```python
from build123d import *

# Parameters (mm, degrees)
SCHIZZO1_R                   = 55
ESTRUSIONE_ESTRUSIONE1_DEPTH = 47
SCHIZZO2_R                   = 51
TAGLIO_ESTRUSIONE1_DEPTH     = 44
SCHIZZO3_W                   = 6.7
SCHIZZO3_H                   = 21
ESTRUSIONE_ESTRUSIONE2_DEPTH = 25
SCHIZZO9_R                   = 1.75
TAGLIO_ESTRUSIONE2_DEPTH     = 12
TAGLIO_ESTRUSIONE3_START     = 45
SCHIZZO10_W                  = 12
SCHIZZO10_H                  = 6
TAGLIO_ESTRUSIONE3_DEPTH     = 67
SCHIZZO12_R                  = 2.2
TAGLIO_ESTRUSIONE4_DEPTH     = 90.364422451
SCHIZZO13_R                  = 4.5
ESTRUSIONE_ESTRUSIONE4_DEPTH = 44
SCHIZZO14_R                  = 1.25
TAGLIO_ESTRUSIONE6_DEPTH     = 12


with BuildPart() as part:
    # Schizzo1 → Estrusione-Estrusione1 (new body)
    with BuildSketch(Plane(origin=(0, 0, 0), x_dir=(1, 0, 0), z_dir=(0, 1, 0))):
        with Locations(Location((0, 0, 0), (0, 0, 270))):
            Circle(SCHIZZO1_R)
    extrude(amount=ESTRUSIONE_ESTRUSIONE1_DEPTH)

    # Schizzo2 → Taglio-Estrusione1 (cut)
    with BuildSketch(Plane(origin=(0, 47, 0), x_dir=(1, 0, 0), z_dir=(0, 1, 0))):
        with Locations(Location((0, 0, 0), (0, 0, 270))):
            Circle(SCHIZZO2_R)
    extrude(amount=-TAGLIO_ESTRUSIONE1_DEPTH, mode=Mode.SUBTRACT)

    # Schizzo3 → Estrusione-Estrusione2 (add)
    with BuildSketch(Plane(origin=(0, 3, 0), x_dir=(1, 0, 0), z_dir=(0, 1, 0))):
        with Locations((-13.65, 0)):
            Rectangle(SCHIZZO3_W, SCHIZZO3_H)
        with Locations((34.65, 0)):
            Rectangle(SCHIZZO3_W, SCHIZZO3_H)
    extrude(amount=ESTRUSIONE_ESTRUSIONE2_DEPTH)

    # Schizzo9 → Taglio-Estrusione2 (cut)
    with BuildSketch(Plane(origin=(0, 28, 0), x_dir=(1, 0, 0), z_dir=(0, 1, 0))):
        with Locations(Location((-13.25, 5, 0), (0, 0, 270))):
            Circle(SCHIZZO9_R)
        with Locations(Location((-13.25, -5, 0), (0, 0, 90))):
            Circle(SCHIZZO9_R)
        with Locations(Location((34.25, 5, 0), (0, 0, 270))):
            Circle(SCHIZZO9_R)
        with Locations(Location((34.25, -5, 0), (0, 0, 90))):
            Circle(SCHIZZO9_R)
    extrude(amount=-TAGLIO_ESTRUSIONE2_DEPTH, mode=Mode.SUBTRACT)

    # Schizzo10 → Taglio-Estrusione3 (cut)
    with BuildSketch(Plane(origin=(0, 0, 0), x_dir=(0, 0, -1), z_dir=(1, 0, 0)).offset(TAGLIO_ESTRUSIONE3_START)):
        with Locations((0, 9)):
            Rectangle(SCHIZZO10_W, SCHIZZO10_H)
    extrude(amount=TAGLIO_ESTRUSIONE3_DEPTH, mode=Mode.SUBTRACT)

    # Schizzo12 → Taglio-Estrusione4 (cut, through all)
    with BuildSketch(Plane(origin=(0, 3, 0), x_dir=(1, 0, 0), z_dir=(0, 1, 0))):
        with Locations(Location((-28.28, 28.28, 0), (0, 0, 270))):
            Circle(SCHIZZO12_R)
        with Locations(Location((28.28, 28.28, 0), (0, 0, 270))):
            Circle(SCHIZZO12_R)
        with Locations(Location((28.28, -28.28, 0), (0, 0, 270))):
            Circle(SCHIZZO12_R)
        with Locations(Location((-28.28, -28.28, 0), (0, 0, 270))):
            Circle(SCHIZZO12_R)
    extrude(amount=-TAGLIO_ESTRUSIONE4_DEPTH, mode=Mode.SUBTRACT)

    # Schizzo13 → Estrusione-Estrusione4 (add)
    with BuildSketch(Plane(origin=(0, 3, 0), x_dir=(1, 0, 0), z_dir=(0, 1, 0))):
        with Locations((0, 47)):
            Circle(SCHIZZO13_R)
        with Locations((40.703193978, -23.5)):
            Circle(SCHIZZO13_R)
        with Locations((-40.703193978, -23.5)):
            Circle(SCHIZZO13_R)
    extrude(amount=ESTRUSIONE_ESTRUSIONE4_DEPTH)

    # Schizzo14 → Taglio-Estrusione6 (cut)
    with BuildSketch(Plane(origin=(0, 47, 0), x_dir=(1, 0, 0), z_dir=(0, 1, 0))):
        with Locations(Location((0, 47, 0), (0, 0, 270))):
            Circle(SCHIZZO14_R)
        with Locations(Location((40.703193978, -23.5, 0), (0, 0, 270))):
            Circle(SCHIZZO14_R)
        with Locations(Location((-40.703193978, -23.5, 0), (0, 0, 270))):
            Circle(SCHIZZO14_R)
    extrude(amount=-TAGLIO_ESTRUSIONE6_DEPTH, mode=Mode.SUBTRACT)


solid = part.part
```
For this review, take the finished solid that the model builds, in its own axes (mm). A direction names the side the tool comes from. Coordinates: 2 decimals unless noted, no trailing zeros. Order: outer loops, then holes, each group sorted by start corner. A loop starts at its lowest first (then second) coordinate and runs counter-clockwise, first axis right, second up. Notation, with made-up numbers: (84, -35) - (91, -35) arc R21 ccw to (91, -8) - close; hole circle Ø5 at (-8.75, -33). An arc over 180 degrees is marked (long way). Answer as a JSON object with one key per item and string values. Group by question number.
1. We need section B-B on x = 28.28. State the section outline as (y, z) points.
2. We need section D-D on x = -13.25. State the section outline as (y, z) points, then the cut area to 3 significant figures.
3. We need section A-A on y = 22. State the section outline as (x, z) points.
4. For faces 3 (the flat face through (1, 3, -1)), 4 (the flat face through (53, 6, 0)), 5 (the cylindrical face through (-29.123, 1.521, -26.248)), list the 3-axis set-ups (+Z, -Z, +X, -X, +Y, -Y) from which the entire face can be reached by the end or side of a thin tool; tool diameter is ignored.
5. For probe 1 along Z at (x, y) = (34, 25); probe 2 along X at (y, z) = (11.5, -10); probe 3 along X at (y, z) = (1.55, 28.28), list the stretches that pass through material, from the lowest coordinate up.
6. The part is to be moulded in two halves that separate along X. For faces 1 (the flat face through (36.41, 47, 24.19)), 2 (the flat face through (-14, 15, 10.5)), say which applies: pulls with the +X half, pulls with the -X half, needs draft (parallel to the pull), parting line crosses it, or undercut.
7. We need section C-C on z = 34.5. State the section outline as (x, y) points.
8. Clearance check with flat-ended pins moving along their axes: P1, Ø3, axis at x = -30.5, y = 15, coming from the -Z side; P2, Ø2, axis at y = 24, z = 42, coming from the -X side; P3, Ø1, axis at x = 4, y = 35, coming from the -Z side. State where each tip first meets the part, or that it passes through.
Final values:
{
 "1": {"outline": "(0, -47.17) - (47, -47.17) - (47, -42.44) - (3, -42.44) - (3, -30.48) - (0, -30.48) - close; (0, -26.08) - (3, -26.08) - (3, 26.08) - (0, 26.08) - close; (0, 30.48) - (3, 30.48) - (3, 42.44) - (47, 42.44) - (47, 47.17) - (0, 47.17) - close"},
 "2": {"outline": "(0, -53.38) - (47, -53.38) - (47, -49.25) - (3, -49.25) - (3, -10.5) - (28, -10.5) - (28, -6.75) - (16, -6.75) - (16, -3.25) - (28, -3.25) - (28, 3.25) - (16, 3.25) - (16, 6.75) - (28, 6.75) - (28, 10.5) - (3, 10.5) - (3, 49.25) - (47, 49.25) - (47, 53.38) - (0, 53.38) - close", "area": "1,120 mm²"},
 "3": {"outline": "circle Ø110 at (0, 0); (-17, -10.5) - (-10.3, -10.5) - (-10.3, 10.5) - (-17, 10.5) - close; (31.3, -10.5) - (38, -10.5) - (38, 10.5) - (31.3, 10.5) - close; hole (-45.2, 23.62) arc R51 ccw to (-2.15, -50.95) arc R4.5 cw (long way) to (2.15, -50.95) arc R51 ccw to (45.2, 23.62) arc R4.5 cw (long way) to (43.05, 27.34) arc R51 ccw to (-43.05, 27.34) arc R4.5 cw (long way) to start; hole circle Ø3.5 at (-13.25, -5); hole circle Ø3.5 at (-13.25, 5); hole circle Ø3.5 at (34.25, -5); hole circle Ø3.5 at (34.25, 5)"},
 "4": {"face 3": "+Y", "face 4": "+X", "face 5": "+Y, -Y"},
 "5": {"probe 1": "-43.23 to -38.01, -10.5 to -6.73, -3.27 to 3.27, 6.73 to 10.5, 38.01 to 43.23", "probe 2": "-54.08 to -50.01, -17 to -10.3, 31.3 to 38, 50.01 to 54.08", "probe 3": "-47.17 to -30.48, -26.08 to 26.08, 30.48 to 47.17"},
 "6": {"face 1": "needs draft", "face 2": "undercut"},
 "7": {"outline": "(-42.83, 0) - (42.83, 0) - (42.83, 47) - (37.56, 47) - (37.56, 3) - (-37.56, 3) - (-37.56, 47) - (-42.83, 47) - close"},
 "8": {"P1": "z = -46.73", "P2": "x = -36.66", "P3": "z = -54.89"}
}
